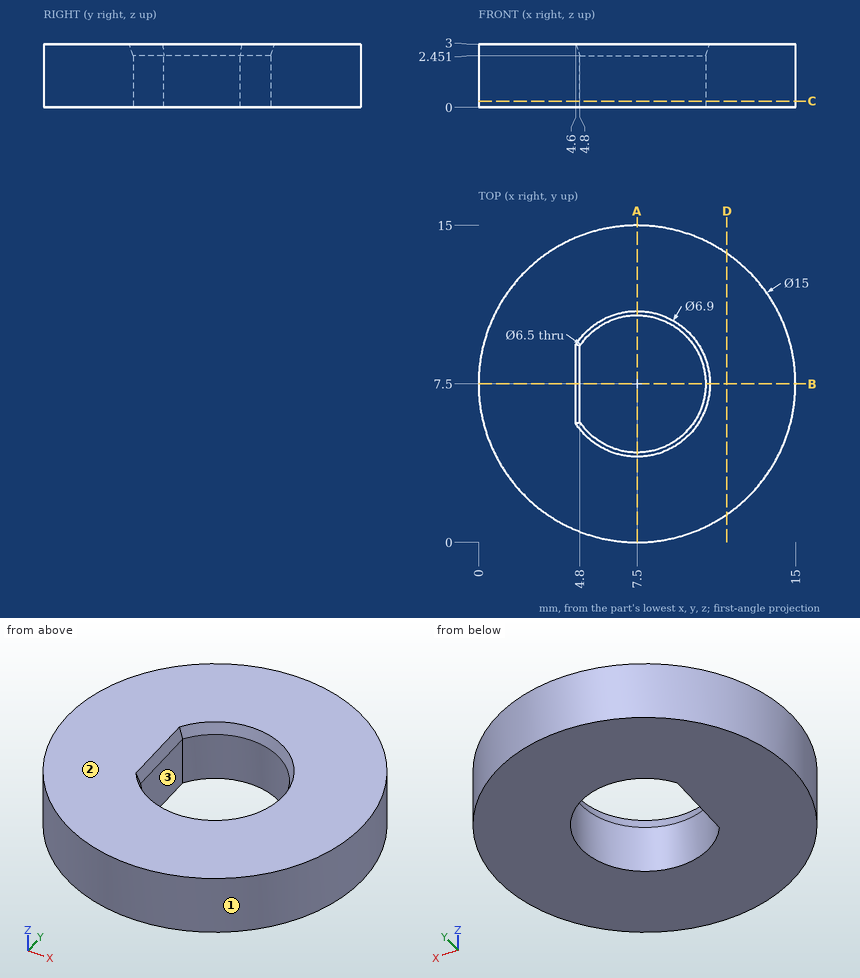
Here's the drawing with two shaded views (mm, measured from the low corner). I have some questions. Give positions to 0.01 mm unless a question says otherwise; leave off trailing zeros. Order: outer loops, then holes, each group sorted by start corner. A loop starts at its lowest first (then second) coordinate and runs counter-clockwise, first axis right, second up. Notation, with made-up numbers: (4, 1.5) -> (11, 1.5) arc R7 ccw to (11, 14.5) -> close; hole circle Ø1 at (64, 6). An arc over 180 degrees is marked (long way). Use a Markdown table: item, result. Add a question column.
Item 1: Imagine slicing it at B-B on y = 7.5. Please give me the cut outline in (x, z).
Item 2: If we mould it in two halves opening along Y, with no side actions, what happens to the marked faces 1, 2 and 3? For each: pulls with the +Y half, pulls with the -Y half, needs draft (parallel to the pull), parting line crosses it, or undercut.
Item 3: Imagine slicing it at C-C on z = 0.3. Please give me the cut outline in (x, y).
Item 4: Will these pins go through, and if not, where does the flat tip stop? pin 1 (1.5 mm diameter, centred on x = 6, y = 6.5, fed in from -Z); pin 2 (1 mm diameter, centred on x = 1.5, z = 2, fed in from +Y); pin 3 (1.5 mm diameter, centred on x = 12.5, z = 2, fed in from -Y).
Item 5: Imagine slicing it at A-A on x = 7.5. Please give me the cut outline in (y, z), plus the area to 3 significant figures.
Item 6: I need wall thicknesses on line 1 (Y direction, x = 7.5, z = 1.05); line 2 (X direction, y = 4.75, z = 0.5) (1 decimal); line 3 (X direction, y = 9.5, z = 1.25). Which ranges of each line are inside material? Lowest first, please.
Item 7: Imagine slicing it at D-D on x = 11.75. Please give me the cut outline in (y, z).
Data:
| question | item | result |
|---|---|---|
| 1 | outline | (0, 0) -> (4.8, 0) -> (4.8, 2.45) -> (4.6, 3) -> (0, 3) -> close; (10.75, 0) -> (15, 0) -> (15, 3) -> (10.95, 3) -> (10.75, 2.45) -> close |
| 2 | face 1 | parting line crosses it |
| 2 | face 2 | needs draft |
| 2 | face 3 | undercut |
| 3 | outline | circle Ø15 at (7.5, 7.5); hole (4.8, 5.69) arc R3.25 ccw (long way) to (4.8, 9.31) -> close |
| 4 | pin 1 | passes through |
| 4 | pin 2 | stops at y = 12.6 |
| 4 | pin 3 | stops at y = 1.32 |
| 5 | outline | (0, 0) -> (4.25, 0) -> (4.25, 2.45) -> (4.05, 3) -> (0, 3) -> close; (10.75, 0) -> (15, 0) -> (15, 3) -> (10.95, 3) -> (10.75, 2.45) -> close |
| 5 | area | 25.4 mm² |
| 6 | line 1 | y = 0 to 4.25, 10.75 to 15 |
| 6 | line 2 | x = 0.5 to 5.8, 9.2 to 14.5 |
| 6 | line 3 | x = 0.27 to 4.94, 10.06 to 14.73 |
| 7 | outline | (1.32, 0) -> (13.68, 0) -> (13.68, 3) -> (1.32, 3) -> close |
